For this review, take the finished solid that the model builds, in its own axes (mm). Round coordinates to 2 decimals unless told otherwise and drop trailing zeros. Order: outer loops, then holes, each group sorted by start corner. A loop starts at its lowest first (then second) coordinate and runs counter-clockwise, first axis right, second up. Notation, with made-up numbers: (37.25, 47) -> (79.25, 47) arc R19 cw to (79.25, 57) -> close; hole circle Ø9 at (87.25, 59.25). An arc over 180 degrees is marked (long way). Put each result on its own line as item: value. Start each with the question number.
```python
from build123d import *

# Parameters (mm, degrees)
F0_W     = 125
F0_H     = 125
F0_R     = 37.5
F1_DEPTH = 2
F2_R     = 3.5
F3_DEPTH = 2.001
F4_R     = 10


with BuildPart() as f1:
    # F0 (on Top) → F1 (new body)
    with BuildSketch(Plane.XY):
        Rectangle(F0_W, F0_H)
        Circle(F0_R, mode=Mode.SUBTRACT)
    extrude(amount=F1_DEPTH)

    # F2 (on Top) → F3 (cut, through all)
    with BuildSketch(Plane.XY):
        with Locations((-51.25, 51.25)):
            Circle(F2_R)
        with Locations((51.25, 51.25)):
            Circle(F2_R)
        with Locations((-51.25, -51.25)):
            Circle(F2_R)
        with Locations((51.25, -51.25)):
            Circle(F2_R)
        with Locations((-32.5, 32.5)):
            Circle(F2_R)
        with Locations((32.5, 32.5)):
            Circle(F2_R)
        with Locations((-32.5, -32.5)):
            Circle(F2_R)
        with Locations((32.5, -32.5)):
            Circle(F2_R)
    extrude(amount=F3_DEPTH, mode=Mode.SUBTRACT)

    # F4
    f4_edges = [f1.edges().sort_by_distance(p)[0] for p in [
        (62.5, -62.5, 1),
        (62.5, 62.5, 1),
        (-62.5, -62.5, 1),
        (-62.5, 62.5, 1),
    ]]
    fillet(f4_edges, radius=F4_R)


solid = f1.part
```
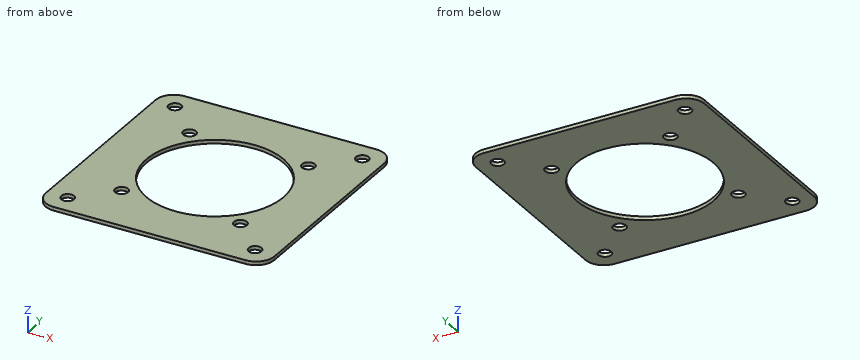
Item 1: Consider section C-C, the plane y = -32.5. Write out the cut boundary in (x, z), plus the area to 3 significant figures.
Item 2: Insertion check: pin 1 Ø9 at (x, y) = (-32.5, 32.5) entering from -Z; pin 2 Ø6.5 at (x, y) = (32.5, 32.5) entering from +Z. Each pin has a flat end and moves straight along its axis. Give the tip position at first contact, or say it passes through.
Item 3: Consider section B-B, the plane z = 1.5. Count the separate pieces of the cut face and the enclosed holes in it, plus the area to 3 significant figures.
Item 4: For L1, parallel to X at y = -51.25, z = 0.85; L2, parallel to X at y = 49.5, z = 1.9, list the stretches that pass through material, from the lowest coordinate up.
Item 5: Consider section D-D, the plane y = 13. Write out the cut boundary in (x, z).
Item 6: Consider section A-A, the plane x = 0. Write out the cut boundary in (y, z), plus the area to 3 significant figures.
Evaluation:
1. outline: (-62.5, 0) -> (-36, 0) -> (-36, 2) -> (-62.5, 2) -> close; (-29, 0) -> (-18.71, 0) -> (-18.71, 2) -> (-29, 2) -> close; (18.71, 0) -> (29, 0) -> (29, 2) -> (18.71, 2) -> close; (36, 0) -> (62.5, 0) -> (62.5, 2) -> (36, 2) -> close
1. area: 147 mm^2
2. pin 1: stops at z = 0
2. pin 2: passes through
3. separate pieces: 1
3. enclosed holes: 9
3. area: 10,800 mm^2
4. L1: x = -62.5 to -54.75, -47.75 to 47.75, 54.75 to 62.5
4. L2: x = -62.5 to -54.28, -48.22 to 48.22, 54.28 to 62.5
5. outline: (-62.5, 0) -> (-35.17, 0) -> (-35.17, 2) -> (-62.5, 2) -> close; (35.17, 0) -> (62.5, 0) -> (62.5, 2) -> (35.17, 2) -> close
6. outline: (-62.5, 0) -> (-37.5, 0) -> (-37.5, 2) -> (-62.5, 2) -> close; (37.5, 0) -> (62.5, 0) -> (62.5, 2) -> (37.5, 2) -> close
6. area: 100 mm^2
